The model under review builds one solid part; all positions refer to its coordinate system, in mm. Coordinates: 2 decimals unless noted, no trailing zeros. Write each loop counter-clockwise with the first axis right and the second up, starting at its lowest first coordinate (ties: lowest second). Pieces come first, ordered by that corner, then holes. Notation, with made-up numbers: (51.5, -35) - (76.5, -35) arc R16 cw to (76.5, -8) - close; hole circle Ø3 at (-19.5, -35.5). An arc over 180 degrees is marked (long way). Put each result on its own line as item: value.
Autodesk Inventor part; units mm, degrees
ref_plane "YZ Plane" through (0, 0, 0) normal (1, 0, 0) x (0, 1, 0)
ref_plane "XZ Plane" through (0, 0, 0) normal (0, 1, 0) x (-1, 0, 0)
ref_plane "XY Plane" through (0, 0, 0) normal (0, 0, 1) x (1, 0, 0)
sketch "Sketch4" plane through (0, 0, 0) normal (0, 1, 0) x (-1, 0, 0)
  circle A0 centre (0, 0) radius 6 construction
  circle A1 centre (0, 0) radius 20 construction
  line L0 (0, 0) -> (-19.8904, -2.0906) construction
  line L1 (0, 0) -> (-19.8904, 2.0906) construction
  line L2 (28, 0) -> (-28, 0)
  arc A2 (-19.8904, 2.0906) -> (-19.8904, -2.0906) centre (0, 0) ccw
  line L3 (-19.8904, 2.0906) -> (-5.9671, 0.6272)
  line L4 (-19.8904, -2.0906) -> (-5.9671, -0.6272)
  arc A3 (-5.9671, 0.6272) -> (-5.9671, -0.6272) centre (0, 0) ccw
  dimension "d38" = 12
  dimension "d39" = 40
  dimension "d41" = 6
  dimension "d42" = 6
extrude "Extrusion5" add sketch "Sketch4" along normal blind 0.1
pattern_circular "Circular Pattern1" count 12 over 360 about axis through (0, -10, 0) along (0, 1, 0) of "Extrusion5"
sketch "Sketch5" plane through (0, 0.1, 0) normal (0, 1, 0) x (1, 0, 0)
  arc A0 (5.4813, 2.4404) -> (4.8541, 3.5267) centre (0, 0) ccw
  arc A1 (5.9671, -0.6272) -> (5.9671, 0.6272) centre (0, 0) ccw
  circle A2 centre (0, 0) radius 6
  circle A3 centre (0, 0) radius 5
  point P0 (4.8541, 3.5267)
  point P1 (5.9671, 0.6272)
  point P2 (5.4813, 2.4404)
  dimension "d48" = 1
extrude "Extrusion6" add sketch "Sketch5" against normal blind 0.1
sketch "Sketch7" plane through (0, 0.1, 0) normal (0, 1, 0) x (1, 0, 0)
  circle A0 centre (0, 0) radius 19 construction
  point P0 (18.974, 0.9944)
  point P1 (19, 0)
  dimension "d55" = 38
  dimension "d56" = 3
hole "Hole1" at (18.974, 0.1, -0.9944) direction (0, -1, 0) diameter 0.7 end through all
pattern_circular "Circular Pattern2" count 3 over 360 about axis through (0, -10, 0) along (0, 1, 0) of "Hole1"
sketch "Sketch8" plane through (0, 0.1, 0) normal (0, 1, 0) x (1, 0, 0)
  circle A0 centre (0, 0) radius 2.5 construction
  circle A1 centre (0, 0) radius 5
  line L0 (5, 0) -> (3, 0)
  line L1 (3, 0) -> (3, 0.5)
  line L2 (3, 0.5) -> (5, 0.5)
  line L3 (5, 0.5) -> (5, 0)
  line L4 (5, 0) -> (3, 0)
  line L5 (3, 0) -> (3, -0.5)
  line L6 (3, -0.5) -> (5, -0.5)
  line L7 (5, -0.5) -> (5, 0)
  circle A2 centre (3, 0) radius 0.5
  circle A3 centre (3, 0) radius 0.25
  point P0 (4.9749, -0.5)
  point P1 (4.9749, 0.5)
  dimension "d67" = 5
  dimension "d68" = 2
  dimension "d69" = 0.5
  dimension "d70" = 0.5
  dimension "d71" = 0.5
extrude "Extrusion8" add sketch "Sketch8" against normal blind 0.1 contours L0 A2 L2 A1 | A1 L6 A2 L0 | A2 L5 A3 L0 | L0 A3 L1 A2 | L1 A3 L5 A2
fillet "Fillet5" radius 0.2 2 edges at (5.9671, 0.05, 0.6272) (5.9671, 0.05, -0.6272)
pattern_circular "Circular Pattern3" count 12 over 360 about axis through (0, 0.1, 0) along (0, -1, 0) of "Fillet5"
fillet "Fillet6" radius 0.2 2 edges at (4.9749, 0.05, -0.5) (4.9749, 0.05, 0.5)
equation "\"d42\" = d41"
properties part number "torsosc-electrode-pcb-cu" material "Copper"
1. Consider section A-A on x = 0. State the section outline as (y, z) points, plus the area to 3 significant figures.
Determined:
outline: (0, -20) - (0.1, -20) - (0.1, -5) - (0, -5) - close; (0, 5) - (0.1, 5) - (0.1, 20) - (0, 20) - close
area: 3.00 mm^2
2. For pin 1 Ø4 at (x, z) = (-8, 12.5) entering from -Y, flat-tipped, find the tip position at first contact; note if it passes through.
Determined:
pin 1: stops at y = 0
3. Consider section D-D on z = -7. State the section outline as (x, y) points, plus the area to 3 significant figures.
Determined:
outline: (-15.72, 0) - (-9.63, 0) - (-9.63, 0.1) - (-15.72, 0.1) - close; (-5.09, 0) - (-3.12, 0) - (-3.12, 0.1) - (-5.09, 0.1) - close; (-0.74, 0) - (0.74, 0) - (0.74, 0.1) - (-0.74, 0.1) - close; (3.12, 0) - (5.09, 0) - (5.09, 0.1) - (3.12, 0.1) - close; (9.63, 0) - (15.72, 0) - (15.72, 0.1) - (9.63, 0.1) - close
area: 1.76 mm^2
4. Consider section B-B on x = 14.5. State the section outline as (y, z) points, plus the area to 3 significant figures.
Determined:
outline: (0, -10.53) - (0.1, -10.53) - (0.1, -6.46) - (0, -6.46) - close; (0, -1.52) - (0.1, -1.52) - (0.1, 1.52) - (0, 1.52) - close; (0, 6.46) - (0.1, 6.46) - (0.1, 10.53) - (0, 10.53) - close
area: 1.12 mm^2
5. To check wall thickness, follow probe 1 along X at (y, z) = (0.05, -8); probe 2 along Z at (x, y) = (6, 0.05); probe 3 along Z at (x, y) = (16, 0.05). State the ranges of each line that lie inside material, in increasing order.
Determined:
probe 1: x = -17.97 to -11.01, -5.81 to -3.56, -0.84 to 0.84, 3.56 to 5.81, 11.01 to 17.97
probe 2: z = -13.48 to -8.26, -4.36 to -2.67, -0.71 to 0.71, 2.67 to 4.36, 8.26 to 13.48
probe 3: z = -11.62 to -7.12, -1.68 to 1.68, 7.12 to 11.62
6. Consider section C-C on z = -14. State the section outline as (x, y) points.
Determined:
outline: (-10.17, 0) - (-6.23, 0) - (-6.23, 0.1) - (-10.17, 0.1) - close; (-1.47, 0) - (1.47, 0) - (1.47, 0.1) - (-1.47, 0.1) - close; (6.23, 0) - (10.17, 0) - (10.17, 0.1) - (6.23, 0.1) - close
